The model under review builds one solid part; all positions refer to its coordinate system, in mm. Face numbers are marked on the shaded views. A direction names the side the tool comes from. Give positions to 0.01 mm unless a question says otherwise; leave off trailing zeros. Write each loop counter-clockwise with the first axis right and the second up, starting at its lowest first coordinate (ties: lowest second). Pieces come first, ordered by that corner, then holes. Notation, with made-up numbers: (51, 66.25) - (83, 66.25) arc R20 cw to (83, 89.25) - close; hole circle Ø2 at (-21, 25). An arc over 180 degrees is marked (long way). Write item = value, one per line.
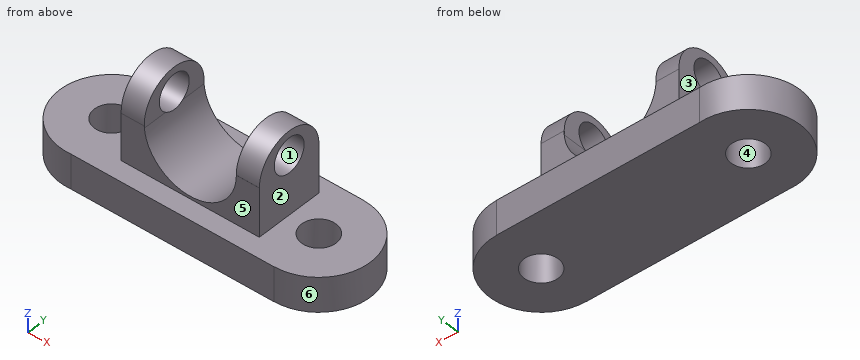
```python
from build123d import *

# Parameters (mm, degrees)
F0_R      = 12.7
F1_DEPTH  = 25.4
F2_W      = 101.6
F2_H      = 50.8
F3_DEPTH  = 35.814
F4_R      = 33.90667
F5_DEPTH  = 57.658
F6_R      = 25.439731
F7_DEPTH  = 17.018
F8_R      = 25.356047
F9_DEPTH  = 17.018
F10_R     = 12.738172
F11_DEPTH = 121.666


with BuildPart() as f1:
    # F0 (on Top) → F1 (new body)
    with BuildSketch(Plane.XY):
        with BuildLine():
            Line((65.169431, 28.175565), (-84.167217, 28.175565))
            ThreePointArc((-84.167217, 28.175565), (-125.453522, -9.924435), (-84.167217, -48.024435))
            Line((-84.167217, -48.024435), (65.169431, -48.024435))
            Line((65.169431, -48.024435), (65.169431, -47.909935))
            ThreePointArc((65.169431, -47.909935), (103.154932, -9.924435), (65.169431, 28.061066))
            Line((65.169431, 28.061066), (65.169431, 28.175565))
        make_face()
        with Locations((-87.230569, -9.924435)):
            Circle(F0_R, mode=Mode.SUBTRACT)
        with Locations((65.169431, -9.924435)):
            Circle(F0_R, mode=Mode.SUBTRACT)
    extrude(amount=F1_DEPTH)

    # F2 (on face) → F3 (join)
    with BuildSketch(Plane.XY.offset(25.4)):
        with Locations((-8.578566, -8.613469)):
            Rectangle(F2_W, F2_H)
    extrude(amount=F3_DEPTH)

    # F4 (on face) → F5 (cut)
    with BuildSketch(Plane.XZ.offset(34.013469)):
        with Locations((-8.578566, 61.214)):
            Circle(F4_R)
    extrude(amount=-F5_DEPTH, mode=Mode.SUBTRACT)

    # F6 (on face) → F7 (join)
    with BuildSketch(Plane(origin=(-59.378566, 0, 0), x_dir=(0, -1, 0), z_dir=(-1, 0, 0))):
        with Locations((8.613469, 61.214)):
            Circle(F6_R)
    extrude(amount=-F7_DEPTH)

    # F8 (on face) → F9 (join)
    with BuildSketch(Plane.YZ.offset(42.221434)):
        with Locations((-8.613469, 61.214)):
            Circle(F8_R)
    extrude(amount=-F9_DEPTH)

    # F10 (on face) → F11 (cut)
    with BuildSketch(Plane(origin=(-59.378566, 0, 0), x_dir=(0, -1, 0), z_dir=(-1, 0, 0))):
        with Locations((8.56952, 68.759516)):
            Circle(F10_R)
    extrude(amount=-F11_DEPTH, mode=Mode.SUBTRACT)


solid = f1.part
```
1. Draft analysis for pull direction Y (two halves, no side actions). For the marked faces 4, 5 and 6, state which applies: +Y half, -Y half, draft (parallel to the pull), parting line (faces both ways), or undercut.
Findings below:
face_4 = undercut
face_5 = -Y half
face_6 = parting line
2. Take a section at C-C on x = -78.5. Give the boundary of the cut face in (y, z).
Findings below:
outline = (-48.02, 0) - (-19.15, 0) - (-19.15, 25.4) - (-48.02, 25.4) - close; (-0.7, 0) - (28.18, 0) - (28.18, 25.4) - (-0.7, 25.4) - close
3. For line 1 (Y direction, x = -87.5, z = 17.5); line 2 (X direction, y = -17.5, z = 58.5); line 3 (X direction, y = 1.5, z = 17.5), list the stretches that pass through material, from the lowest coordinate up. Write a range as from..to.
Findings below:
line_1 = -48.15..-22.62, 2.77..28.3
line_2 = -59.38..-42.36, 25.2..42.22
line_3 = -123.71..-92.78, -81.68..59.62, 70.72..101.4
4. Take a section at B-B on y = -7. Give the boundary of the cut face in (x, z).
Findings below:
outline = (-125.34, 0) - (-99.59, 0) - (-99.59, 25.4) - (-125.34, 25.4) - close; (-74.87, 0) - (52.81, 0) - (52.81, 25.4) - (42.22, 25.4) - (42.22, 56.12) - (24.94, 56.12) arc R33.91 cw to (-42.1, 56.12) - (-59.38, 56.12) - (-59.38, 25.4) - (-74.87, 25.4) - close; (-59.38, 81.4) - (-42.36, 81.4) - (-42.36, 86.6) - (-59.38, 86.6) - close; (25.2, 81.4) - (42.22, 81.4) - (42.22, 86.52) - (25.2, 86.52) - close; (77.53, 0) - (103.04, 0) - (103.04, 25.4) - (77.53, 25.4) - close
5. Take a section at D-D on z = 22. Give the boundary of the cut face in (x, y), and give its area (3 significant figures).
Findings below:
outline = (-84.17, -48.02) - (65.17, -48.02) - (65.17, -47.91) arc R37.99 ccw to (65.17, 28.06) - (65.17, 28.18) - (-84.17, 28.18) arc R38.22 ccw (long way) to start; hole circle Ø25.4 at (-87.23, -9.92); hole circle Ø25.4 at (65.17, -9.92)
area = 15,200 mm²
6. Insertion check: P1, Ø15.5, axis at y = -8.57, z = 68.76, coming from the +X side; P2, Ø1.5, axis at x = -51.5, z = 17.5, coming from the +Y side; P3, Ø14, axis at y = 1.5, z = 70, coming from the -X side; P4, Ø1, axis at x = 55, y = 5.5, coming from the +Z side. Each pin has a flat end and moves straight along its axis. Give the tip position at first contact, or say it passes through.
Findings below:
P1 = through
P2 = 28.18
P3 = -59.38
P4 = 25.4
7. Machinability: for the marked faces 1, 2 and 3, which of the approach directions +Z, -Z, +X, -X, +Y, -Y give a long, thin tool a straight path to every point of the face, cutting with its end or side? Answer none if there is none.
Findings below:
face_1 = +X, -X
face_2 = +Z, +X, +Y, -Y
face_3 = +Z, -X, +Y, -Y
8. Take a section at A-A on z = 43.5. Give the boundary of the cut face in (x, y).
Findings below:
outline = (-59.38, -34.01) - (-37.49, -34.01) - (-37.49, 16.79) - (-59.38, 16.79) - close; (20.33, -34.01) - (42.22, -34.01) - (42.22, 16.79) - (20.33, 16.79) - close
